```python
from build123d import *

# Parameters (mm, degrees)
SKETCH1_R           = 1.5
SKETCH1_R_2         = 3
SKETCH1_R_3         = 5
BOSS_EXTRUDE1_DEPTH = 3.175


with BuildPart() as part:
    # Sketch1 → Boss-Extrude1 (new body)
    with BuildSketch(Plane(origin=(0, 0, 0), x_dir=(1, 0, 0), z_dir=(0, 1, 0))):
        Polygon((70, 110.468098835), (450, 110.468098835), (450, 310.468098835), (70, 310.468098835), (0, 310.468098835), (0, 110.468098835), align=None)
        with Locations(Location((410, 225.468098835, 0), (0, 0, 270))):
            Circle(SKETCH1_R, mode=Mode.SUBTRACT)
        with Locations(Location((410, 195.468098835, 0), (0, 0, 270))):
            Circle(SKETCH1_R, mode=Mode.SUBTRACT)
        with Locations(Location((10, 260.468098835, 0), (0, 0, 270))):
            Circle(SKETCH1_R_2, mode=Mode.SUBTRACT)
        with Locations(Location((440, 300.468098835, 0), (0, 0, 270))):
            Circle(SKETCH1_R_2, mode=Mode.SUBTRACT)
        with Locations(Location((140, 300.468098835, 0), (0, 0, 270))):
            Circle(SKETCH1_R_2, mode=Mode.SUBTRACT)
        with Locations(Location((290, 300.468098835, 0), (0, 0, 270))):
            Circle(SKETCH1_R_2, mode=Mode.SUBTRACT)
        with Locations(Location((440, 120.468098835, 0), (0, 0, 90))):
            Circle(SKETCH1_R_2, mode=Mode.SUBTRACT)
        with Locations(Location((290, 120.468098835, 0), (0, 0, 90))):
            Circle(SKETCH1_R_2, mode=Mode.SUBTRACT)
        with Locations(Location((140, 120.468098835, 0), (0, 0, 90))):
            Circle(SKETCH1_R_2, mode=Mode.SUBTRACT)
        with Locations(Location((10, 160.468098835, 0), (0, 0, 90))):
            Circle(SKETCH1_R_2, mode=Mode.SUBTRACT)
        with Locations(Location((35, 210.468098835, 0), (0, 0, 270))):
            Circle(SKETCH1_R_3, mode=Mode.SUBTRACT)
        with Locations(Location((140, 211.808399399, 0), (0, 0, 270))):
            Circle(SKETCH1_R_3, mode=Mode.SUBTRACT)
    extrude(amount=BOSS_EXTRUDE1_DEPTH)


solid = part.part
```
Could you check a few things on this model? Use its own coordinates, in mm. Round coordinates to 2 decimals unless told otherwise and drop trailing zeros. Order: outer loops, then holes, each group sorted by start corner. A loop starts at its lowest first (then second) coordinate and runs counter-clockwise, first axis right, second up. Notation, with made-up numbers: M 86,62.5 L 139,62.5 A8 ccw 139,75.5 Z; hole C 30.5,0.25 d11. An arc over 180 degrees is marked long. One line per question, with ' | ' between items. Start each with the question number.
(1) Please list where these lines run through material, in increasing order: line 1 along X through (y, z) = (0.7, -120); line 2 along Z through (x, y) = (440, 1.1); line 3 along Z through (x, y) = (410, 1.3).
(2) Suppose I cut it at A-A on x = 35. List the corners of the cut face in (y, z) for me (3 decimals).
(3) Thinking about a two-plate mould opening in Z: for faces 1 (the face through (135.564, 1.565, -209.501)), 2 (the face through (222, 0, -212)), which applies, +Z half, -Z half, draft (parallel to the pull), parting line (faces both ways), or undercut?
Geometry results:
1) line 1: 0 to 137.04, 142.96 to 287.04, 292.96 to 437.04, 442.96 to 450 | line 2: -310.47 to -303.47, -297.47 to -123.47, -117.47 to -110.47 | line 3: -310.47 to -226.97, -223.97 to -196.97, -193.97 to -110.47
2) outline: M 0,-310.468 L 3.175,-310.468 L 3.175,-215.468 L 0,-215.468 Z; M 0,-205.468 L 3.175,-205.468 L 3.175,-110.468 L 0,-110.468 Z
3) face 1: undercut | face 2: draft
